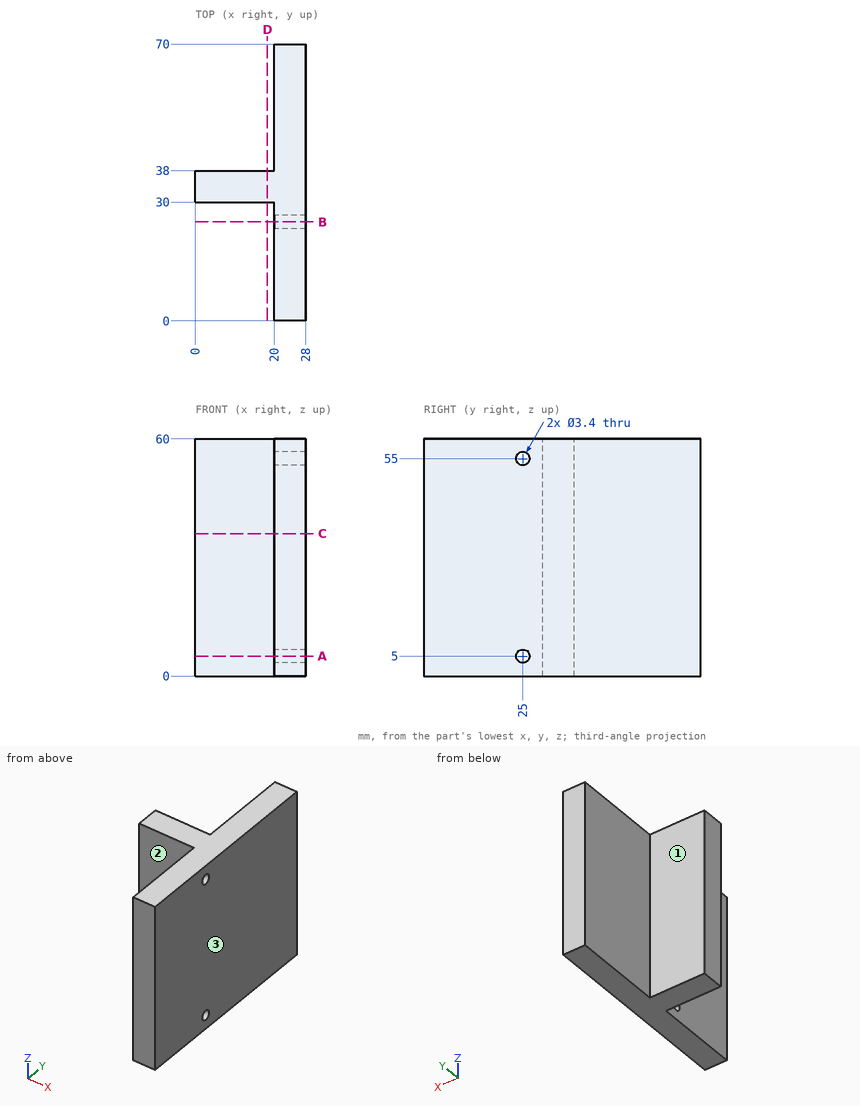
Geometry check sheet. Reference: drawing and pictorial views, mm from the part's lowest x, y, z. A direction names the side the tool comes from. Give positions to 0.01 mm unless a question says otherwise; leave off trailing zeros. Order: outer loops, then holes, each group sorted by start corner. A loop starts at its lowest first (then second) coordinate and runs counter-clockwise, first axis right, second up.
1. Section check A-A, the plane z = 5. Enter the section's corners in (x, y), and give its area (3 significant figures).
2. Section check D-D, the plane x = 18.25. Enter the section's corners in (y, z), and give its area (3 significant figures).
3. Gauge pin test, flat ends, axial feed: pin 1 Ø12 at (x, z) = (6, 16.5) entering from -Y; pin 2 Ø16 at (x, z) = (7, 39) entering from +Y; pin 3 Ø5 at (y, z) = (27, 39) entering from -X. Record the tip position at first contact, or that the pin passes through.
4. Section check C-C, the plane z = 36. Enter the section's corners in (x, y), and give its area (3 significant figures).
5. Section check B-B, the plane y = 25. Enter the section's corners in (x, z), and give its area (3 significant figures).
6. Thickness scan on L1, parallel to Z at x = 24, y = 25; L2, parallel to Y at x = 25.25, z = 5; L3, parallel to Y at x = 17.25, z = 47. Record the ranges inside material, lowest first.
7. Access from +Z, -Z, +X, -X, +Y, -Y to the whole of each face (thin tool, end or side, straight path). Record for the marked faces 1, 2 and 3.
Values follow:
1. outline: (0, 30) - (20, 30) - (20, 26.7) - (28, 26.7) - (28, 70) - (20, 70) - (20, 38) - (0, 38) - close; (20, 0) - (28, 0) - (28, 23.3) - (20, 23.3) - close
1. area: 693 mm2
2. outline: (30, 0) - (38, 0) - (38, 60) - (30, 60) - close
2. area: 480 mm2
3. pin 1: stops at y = 30
3. pin 2: stops at y = 38
3. pin 3: stops at x = 20
4. outline: (0, 30) - (20, 30) - (20, 0) - (28, 0) - (28, 70) - (20, 70) - (20, 38) - (0, 38) - close
4. area: 720 mm2
5. outline: (20, 0) - (28, 0) - (28, 3.3) - (20, 3.3) - close; (20, 6.7) - (28, 6.7) - (28, 53.3) - (20, 53.3) - close; (20, 56.7) - (28, 56.7) - (28, 60) - (20, 60) - close
5. area: 426 mm2
6. L1: z = 0 to 3.3, 6.7 to 53.3, 56.7 to 60
6. L2: y = 0 to 23.3, 26.7 to 70
6. L3: y = 30 to 38
7. face 1: +Z, -Z, -X, +Y
7. face 2: +Z, -Z, -X, -Y
7. face 3: +Z, -Z, +X, +Y, -Y
